Read the model definition and answer for the solid it produces. Units are mm, in the model's axes. A direction names the side the tool comes from. Coordinates: 2 decimals unless noted, no trailing zeros. Write each loop counter-clockwise with the first axis right and the second up, starting at its lowest first coordinate (ties: lowest second). Pieces come first, ordered by that corner, then holes.
from build123d import *

# Parameters (mm, degrees)
SKETCH1_R               = 20
SKETCH1_R_2             = 15
BOSS_EXTRUDE1_DEPTH     = 20
CUT_EXTRUDE2_DEPTH      = 21
CUT_EXTRUDE2_DEPTH_BACK = 1
BOSS_EXTRUDE16_DEPTH    = 10
CIRPATTERN2_COUNT       = 6


with BuildPart() as part:
    # Sketch1 → Boss-Extrude1 (new body)
    with BuildSketch(Plane.XY):
        Circle(SKETCH1_R)
        Circle(SKETCH1_R_2, mode=Mode.SUBTRACT)
    extrude(amount=BOSS_EXTRUDE1_DEPTH)

    # Sketch5 → Cut-Extrude2 (cut, two sides)
    with BuildSketch(Plane.XY) as cut_extrude2_sk:
        with BuildLine():
            Line((-4, -17.293255897), (0, -17.293255897))
            Line((0, -17.293255897), (4, -17.293255897))
            Line((4, -17.293255897), (4, -14.456832295))
            ThreePointArc((4, -14.456832295), (0, -15), (-4, -14.456832295))
            Line((-4, -14.456832295), (-4, -17.293255897))
        make_face()
    extrude(amount=CUT_EXTRUDE2_DEPTH, mode=Mode.SUBTRACT)
    extrude(cut_extrude2_sk.sketch, amount=-CUT_EXTRUDE2_DEPTH_BACK, mode=Mode.SUBTRACT)

    # Sketch18 → Boss-Extrude16 (add)
    with BuildSketch(Plane.XY.offset(5)):
        with BuildLine():
            Line((0, 27), (0, 20))
            ThreePointArc((0, 20), (6.296505517, 18.982992869), (11.952651932, 16.035401828))
            Line((11.952651932, 16.035401828), (0, 27))
        make_face()
    boss_extrude16 = extrude(amount=BOSS_EXTRUDE16_DEPTH)

    # CirPattern2: Boss-Extrude16 ×6 about axis
    cirpattern2_axis = Axis((0, 0, 0), (0, 0, 1))
    for i in range(1, CIRPATTERN2_COUNT):
        add(boss_extrude16.rotate(cirpattern2_axis, i * 360 / CIRPATTERN2_COUNT))


solid = part.part
Item 1: Determine the mould class of faces 4 (the flat face through (-6.06, -21.44, 9.93)), 5 (the flat face through (4, -16, 10)), 6 (the flat face through (20.39, -11.77, 9.93)), 7 (the flat face through (0, 24, 10)) for opening direction Y: +Y half, -Y half, draft (parallel to the pull), parting line (faces both ways), or undercut.
Item 2: Given pin 1 (2 mm diameter, centred on x = -3, z = 4, fed in from +Y); pin 2 (3.5 mm diameter, centred on y = 22.5, z = 9, fed in from -X); pin 3 (2.5 mm diameter, centred on x = 17.5, y = -16, fed in from +Z); pin 4 (2.5 mm diameter, centred on x = 12, y = -14.5, fed in from -Z), each flat-ended and moving along its own axis, determine where each tip first touches the part or whether it passes through.
Item 3: The part is cut by section D-D (y = -19). Give the vertices of the cut face in (x, z) (3 decimals).
Item 4: The part is cut by section A-A (z = 9.25). Give the vertices of the cut face in (x, y).
Item 5: Find the intervals of material crossed by probe 1 along Y at (x, z) = (13.5, 13.75); probe 2 along X at (y, z) = (0, 9); probe 3 along Y at (x, z) = (3.5, 13.25), in increasing order.
Item 6: The part is cut by section C-C (x = 11). Give the vertices of the cut face in (y, z).
Item 7: For faces 1 (the flat face through (-17, 14, 15)), 2 (the flat face through (-20.39, 11.77, 9.93)), 3 (the cylindrical face through (18.475, -7.66, 9.86)), determine the directions among +Z, -Z, +X, -X, +Y, -Y from which every point of the face is accessible in a straight line to the end or side of a thin tool.
Item 8: The part is cut by section B-B (y = -4). Give the vertices of the cut face in (x, z).
Answer:
1. face 4: -Y half
1. face 5: undercut
1. face 6: undercut
1. face 7: draft
2. pin 1: stops at y = 19.9
2. pin 2: stops at x = 0
2. pin 3: stops at z = 15
2. pin 4: stops at z = 0
3. outline: (-8.721, 5) - (-6.245, 5) - (-6.245, 0) - (6.245, 0) - (6.245, 20) - (-6.245, 20) - (-6.245, 15) - (-8.721, 15) - close
4. outline: (-23.38, -13.5) - (-17.32, -10) arc R20 ccw to (-11.95, -16.04) - (0, -27) - (0, -20) arc R20 ccw to (7.91, -18.37) - (23.38, -13.5) - (17.32, -10) arc R20 ccw to (19.86, -2.33) - (23.38, 13.5) - (17.32, 10) arc R20 ccw to (11.95, 16.04) - (0, 27) - (0, 20) arc R20 ccw to (-7.91, 18.37) - (-23.38, 13.5) - (-17.32, 10) arc R20 ccw to (-19.86, 2.33) - close; hole (-4, -17.29) - (4, -17.29) - (4, -14.46) arc R15 ccw (long way) to (-4, -14.46) - close
5. probe 1: y = -16.61 to -6.54, 6.54 to 14.76
5. probe 2: x = -20.38 to -15, 15 to 20.38
5. probe 3: y = -19.69 to -17.29, 14.59 to 23.79
6. outline: (-17.4, 5) - (-16.7, 5) - (-16.7, 0) - (-10.2, 0) - (-10.2, 20) - (-16.7, 20) - (-16.7, 15) - (-17.4, 15) - close; (10.2, 0) - (16.7, 0) - (16.7, 5) - (16.91, 5) - (16.91, 15) - (16.7, 15) - (16.7, 20) - (10.2, 20) - close
7. face 1: +Z, -X, +Y
7. face 2: +Z, -Z, -X
7. face 3: none
8. outline: (-21.27, 5) - (-19.6, 5) - (-19.6, 0) - (-14.46, 0) - (-14.46, 20) - (-19.6, 20) - (-19.6, 15) - (-21.27, 15) - close; (14.46, 0) - (19.6, 0) - (19.6, 20) - (14.46, 20) - close
